Check sheet for the modelled part. Datum: model origin and axes. Units: mm. A direction names the side the tool comes from. Give positions to 0.01 mm unless a question says otherwise; leave off trailing zeros. Write each loop counter-clockwise with the first axis right and the second up, starting at its lowest first coordinate (ties: lowest second). Pieces come first, ordered by that corner, then holes. Notation, with made-up numbers: M 77,73.5 L 112,73.5 A6 cw 112,80.5 Z; hole C 3,-32 d10. An arc over 180 degrees is marked long. Use CSV: the item, a comma, the result in double quotes. Start each with the question number.
1. Cross-section at C-C, the plane z = -23.75. Enter the section's corners in (x, y).
2. Mould release check, pull along Z, two halves, no side actions. Record for faces 1 (the face through (-37, 16, -20)), 2 (the face through (50.8, 0.7, -22.4)), 3 (the face through (-37, 9, -25)): +Z half, -Z half, draft (parallel to the pull), parting line (faces both ways), or undercut.
3. Scan lines: line 1 (Z direction, x = -49, y = 0.8); line 2 (Z direction, x = 47, y = 4); line 3 (X direction, y = 3.5, z = 25.5). Record each from-to range of solid material in increasing order.
4. Access from +Z, -Z, +X, -X, +Y, -Y to the whole of each face (thin tool, end or side, straight path). Record for faces 4 (the face through (-37, 9, -14.5)), 5 (the face through (44, 8, -5)), 6 (the face through (-43.3, 9, -20)), 7 (the face through (39.8, 8, 0)), 8 (the face through (48.8, 6, 0)).
5. Cross-section at D-D, the plane x = -2.5. Enter the section's corners in (y, z).
6. Cross-section at A-A, the plane y = 6.25. Enter the section's corners in (x, z), and give its area (4 significant figures).
7. Depth check by flat-ended pin: P1, Ø2, axis at x = 42, z = 1.5, coming from the +Y side; P2, Ø7, axis at x = 45.5, y = 10.5, coming from the +Z side; P3, Ø4, axis at x = -35, y = 6, coming from the -Z side; P4, Ø8, axis at x = -22, y = 6, coming from the -Z side. Enter the tip coordinate at first touch or a pass-through.
8. Cross-section at B-B, the plane x = -49. Enter the section's corners in (y, z), and give its area (3 significant figures).
Autodesk Inventor part; units mm, degrees
ref_plane "YZ Plane" through (0, 0, 0) normal (1, 0, 0) x (0, 1, 0)
ref_plane "XZ Plane" through (0, 0, 0) normal (0, 1, 0) x (-1, 0, 0)
ref_plane "XY Plane" through (0, 0, 0) normal (0, 0, 1) x (1, 0, 0)
sketch "스케치1" plane through (0, 0, 0) normal (0, 1, 0) x (-1, 0, 0)
  line L0 (-53.3, 28.5) -> (53.3, 28.5)
  line L1 (53.3, 28.5) -> (53.3, -28.5)
  line L2 (53.3, -28.5) -> (-53.3, -28.5)
  line L3 (-53.3, -28.5) -> (-53.3, 28.5)
  line L4 (-53.3, 28.5) -> (53.3, -28.5) construction
  line L5 (53.3, 28.5) -> (-53.3, -28.5) construction
  circle A0 centre (49, 23.75) radius 2.25
  line L6 (0, 0) -> (18.7645, 0)
  line L7 (0, 0) -> (0, -10.3185)
  circle A1 centre (-49, 23.75) radius 2.25
  circle A2 centre (49, -23.75) radius 2.25
  circle A3 centre (-49, -23.75) radius 2.25
  dimension "d0" = 106.6
  dimension "d1" = 57
  dimension "d2" = 4.5
  dimension "d3" = 47.5
  dimension "d4" = 98
extrude "돌출1" add sketch "스케치1" along normal blind 1.5
sketch "스케치2" plane through (0, 1.5, 0) normal (0, 1, 0) x (1, 0, 0)
  line L0 (-43.3, 14.5) -> (-30.3, 14.5)
  line L1 (-30.3, 14.5) -> (-30.3, 25)
  line L2 (-30.3, 25) -> (-43.3, 25)
  line L3 (-43.3, 25) -> (-43.3, 14.5)
  line L4 (-43.3, 14.5) -> (-30.3, 25) construction
  line L5 (-30.3, 14.5) -> (-43.3, 25) construction
  line L6 (-53.3, 28.5) -> (-53.3, -28.5)
  line L7 (53.3, 28.5) -> (-53.3, 28.5)
  point P0 (0, 0)
  point P1 (-36.8, 19.75)
  dimension "d7" = 10.5
  dimension "d8" = 13
  dimension "d9" = 10
  dimension "d10" = 3.5
extrude "돌출2" add sketch "스케치2" along normal blind 14.5
sketch "스케치3" plane through (0, 1.5, 0) normal (0, 1, 0) x (1, 0, 0)
  line L0 (12.5, -27.5) -> (-12.5, -27.5)
  line L1 (-12.5, -27.5) -> (-12.5, 2.5)
  line L2 (-12.5, 2.5) -> (12.5, 2.5)
  line L3 (12.5, 2.5) -> (12.5, -27.5)
  line L4 (12.5, -27.5) -> (-12.5, 2.5) construction
  line L5 (-12.5, -27.5) -> (12.5, 2.5) construction
  line L6 (-53.3, -28.5) -> (53.3, -28.5)
  point P0 (0, 0)
  point P1 (0, -12.5)
  dimension "d13" = 25
  dimension "d14" = 30
  dimension "d15" = 16
extrude "돌출3" add sketch "스케치3" along normal blind 28
sketch "스케치4" plane through (0, 0, 0) normal (0, 0, 1) x (1, 0, 0)
  line L0 (-53.3, 1.5) -> (53.3, 1.5)
  line L1 (48.8, 1.5) -> (48.8, 11.5)
  line L2 (48.8, 11.5) -> (46.6994, 14.5)
  line L3 (46.6994, 14.5) -> (39.8, 14.5)
  line L4 (39.8, 14.5) -> (39.8, 1.5)
  point P0 (0, 0)
  dimension "d18" = 9
  dimension "d19" = 145
  dimension "d20" = 13
  dimension "d21" = 4.5
  dimension "d22" = 10
extrude "돌출4" add sketch "스케치4" along normal mid plane 10
properties part number "AC-DC컨버터"
Worked answers:
1,outline,"M -53.3,0 L -51.25,0 L -51.25,1.5 L -53.3,1.5 Z; M -46.75,0 L 46.75,0 L 46.75,1.5 L -30.3,1.5 L -30.3,16 L -43.3,16 L -43.3,1.5 L -46.75,1.5 Z; M 51.25,0 L 53.3,0 L 53.3,1.5 L 51.25,1.5 Z"
2,face 1,"draft"
2,face 2,"undercut"
2,face 3,"-Z half"
3,line 1,"z = -28.5 to -26, -21.5 to 21.5, 26 to 28.5"
3,line 2,"z = -5 to 5"
3,line 3,"x = -12.5 to 12.5"
4,face 4,"+Z, +X, -X, +Y"
4,face 5,"-Z, +X, -X, +Y"
4,face 6,"+Z, -Z, -X, +Y"
4,face 7,"+Z, -Z, +Y"
4,face 8,"+Z, -Z, +X, +Y"
5,outline,"M 0,-28.5 L 1.5,-28.5 L 1.5,-2.5 L 29.5,-2.5 L 29.5,27.5 L 1.5,27.5 L 1.5,28.5 L 0,28.5 Z"
6,outline,"M -43.3,-25 L -30.3,-25 L -30.3,-14.5 L -43.3,-14.5 Z; M -12.5,-2.5 L 12.5,-2.5 L 12.5,27.5 L -12.5,27.5 Z; M 39.8,-5 L 48.8,-5 L 48.8,5 L 39.8,5 Z"
6,area,"976.5 mm^2"
7,P1,"stops at y = 14.5"
7,P2,"stops at z = 5"
7,P3,"stops at z = -25"
7,P4,"passes through"
8,outline,"M 0,-28.5 L 1.5,-28.5 L 1.5,-26 L 0,-26 Z; M 0,-21.5 L 1.5,-21.5 L 1.5,21.5 L 0,21.5 Z; M 0,26 L 1.5,26 L 1.5,28.5 L 0,28.5 Z"
8,area,"72.0 mm^2"
